from build123d import *

# Parameters (mm, degrees)
SKETCH1_R           = 1
BOSS_EXTRUDE1_DEPTH = 3
SKETCH2_R           = 0.8
BOSS_EXTRUDE2_DEPTH = 3
FILLET1_R           = 2


with BuildPart() as part:
    # Sketch1 → Boss-Extrude1 (new body)
    with BuildSketch(Plane(origin=(0, 0, 0), x_dir=(1, 0, 0), z_dir=(0, 1, 0))):
        with BuildLine():
            Line((0, -3), (0, -5))
            Line((0, -5), (-15.705, -5))
            Line((-15.705, -5), (-15.705, 7))
            Line((-15.705, 7), (0, 7))
            Line((0, 7), (0, 1))
            ThreePointArc((0, 1), (-2, -1), (0, -3))
        make_face()
        with Locations(Location((-10.705, -1, 0), (0, 0, 270))):
            Circle(SKETCH1_R, mode=Mode.SUBTRACT)
    boss_extrude1 = extrude(amount=BOSS_EXTRUDE1_DEPTH)

    # Sketch2 → Boss-Extrude2 (add)
    with BuildSketch(Plane(origin=(0, 0, -7), x_dir=(-1, 0, 0), z_dir=(0, 0, -1))):
        Polygon((15.705, 3), (15.705, 18), (22.3, 18), (22.3, 38.9), (0, 38.9), (0, 22), (6.5, 22), (6.5, 9), (0, 9), (0, 3), align=None)
        with Locations((20.53, 19.88)):
            Circle(SKETCH2_R, mode=Mode.SUBTRACT)
        with Locations(Location((20.53, 37.02, 0), (0, 0, 180))):
            Circle(SKETCH2_R, mode=Mode.SUBTRACT)
    boss_extrude2 = extrude(amount=-BOSS_EXTRUDE2_DEPTH)

    # Mirror1: Boss-Extrude1, Boss-Extrude2 across plane
    add(boss_extrude1.mirror(Plane(origin=(0, 0, 0), x_dir=(0, 0, 1), z_dir=(1, 0, 0))))
    add(boss_extrude2.mirror(Plane(origin=(0, 0, 0), x_dir=(0, 0, 1), z_dir=(1, 0, 0))))

    # Fillet1
    fillet1_edges = [part.edges().sort_by_distance(p)[0] for p in [
        (0, 3, -4),
        (0, 0, -7),
    ]]
    fillet(fillet1_edges, radius=FILLET1_R)


solid = part.part
Could you check a few things on this model? Use its own coordinates, in mm. A direction names the side the tool comes from. Give positions to 0.01 mm unless a question says otherwise; leave off trailing zeros. Order: outer loops, then holes, each group sorted by start corner. A loop starts at its lowest first (then second) coordinate and runs counter-clockwise, first axis right, second up. Notation, with made-up numbers: M 18.25,56.25 L 44.25,56.25 A24 ccw 44.25,74.25 Z; hole C -23.5,-35.75 d7. An arc over 180 degrees is marked long. One line per question, with ' | ' between items.
1. For faces 1 (the face through (15.705, 5, -5)), 2 (the face through (-6.5, 16, -6)), 3 (the face through (-15.705, 5, -5)), 4 (the face through (0, 3, 4)), which set-ups out of +Z, -Z, +X, -X, +Y, -Y let a thin tool reach every point of the face, with its end or its side?
Results:
face 1: +Z, -Z, +X, -Y | face 2: +Z, -Z | face 3: +Z, -Z, -X, -Y | face 4: +Z, +X, -X, +Y
2. I want a section at A-A (x = 4.5). List the corners of the cut face in (y, z) for me, and give its area (3 significant figures).
Results:
outline: M 0,-5 A2 ccw 2,-7 L 9,-7 L 9,-4 L 5,-4 A2 cw 3,-2 L 3,5 L 0,5 Z; M 22,-7 L 38.9,-7 L 38.9,-4 L 22,-4 Z | area: 105 mm²
3. I want a section at D-D (z = 1). List the corners of the cut face in (x, y) for me (3 decimals).
Results:
outline: M -15.705,0 L -11.705,0 L -11.705,3 L -15.705,3 Z; M -9.705,0 L -2,0 L -2,3 L -9.705,3 Z; M 2,0 L 9.705,0 L 9.705,3 L 2,3 Z; M 11.705,0 L 15.705,0 L 15.705,3 L 11.705,3 Z
4. We'd pull the mould along X, two halves only. Please class faces 5 (the face through (-0.22, 0.57, -6.4)), 6 (the face through (-22.3, 28, -6)), 7 (the face through (6.5, 16, -6)): +X half, -X half, draft (parallel to the pull), parting line (faces both ways), or undercut.
Results:
face 5: draft | face 6: -X half | face 7: undercut
5. I want a section at C-C (y = 19.88). List the corners of the cut face in (x, z) for me, and give its area (3 significant figures).
Results:
outline: M -22.3,-7 L -21.33,-7 L -21.33,-4 L -22.3,-4 Z; M -19.73,-7 L -6.5,-7 L -6.5,-4 L -19.73,-4 Z; M 6.5,-7 L 19.73,-7 L 19.73,-4 L 6.5,-4 Z; M 21.33,-7 L 22.3,-7 L 22.3,-4 L 21.33,-4 Z | area: 85.2 mm²
6. I want a section at B-B (x = 20.53). List the corners of the cut face in (y, z) for me.
Results:
outline: M 18,-7 L 19.08,-7 L 19.08,-4 L 18,-4 Z; M 20.68,-7 L 36.22,-7 L 36.22,-4 L 20.68,-4 Z; M 37.82,-7 L 38.9,-7 L 38.9,-4 L 37.82,-4 Z
7. If I drill on line 1 (X direction, y = 1.3, z = 1) (3 decimals); line 2 (Y direction, x = 20.53, z = -5.7); line 3 (X direction, y = 19.5, z = -6.5), over which ranges is the centre line in solid material (lowest first)?
Results:
line 1: -15.705 to -11.705, -9.705 to -2, 2 to 9.705, 11.705 to 15.705 | line 2: 18 to 19.08, 20.68 to 36.22, 37.82 to 38.9 | line 3: -22.3 to -21.23, -19.83 to -6.5, 6.5 to 19.83, 21.23 to 22.3
8. I'm going to push flat-ended pins straight in: pin 1 (5 mm diameter, centred on y = 4.5, z = 2, fed in from +X) (3 decimals); pin 2 (3.5 mm diameter, centred on x = -2.5, z = 0.5, fed in from +Y); pin 3 (2.5 mm diameter, centred on x = 20.53, y = 37.02, fed in from +Z). Where does each tip first touch, or does it pass through?
Results:
pin 1: x = 15.705 | pin 2: y = 3 | pin 3: z = -4
